Source: three-view drawing plus pictorial views. Frame: mm from the lowest corner of the part. Give positions to 0.01 mm unless a question says otherwise; leave off trailing zeros. Loops run counter-clockwise (first coordinate to the right, second up) from the corner with the lowest first, then second, coordinate; pieces in that order, holes last. Notation, with made-up numbers: M 49.25,-16 L 88.25,-16 A22 cw 88.25,-8 Z; hole C 42.5,23 d8. An arc over 180 degrees is marked long. Answer as a JSON object with one key per item and string values. Group by question number.
1) Section query D-D on x = 84.5. Return loops of the section in (y, z).
2) First-contact query: P1, Ø1, axis at y = 12.5, z = 3.5, coming from the -X side; P2, Ø3, axis at x = 51.6, y = 17.5, coming from the -Z side. Flat tips, straight axial feed; report the tip coordinate or a pass-through.
3) Ray query, L1, parallel to Y at x = 5, z = 4.5; L2, parallel to Y at x = 50.5, z = 4.5; L3, parallel to X at y = 17, z = 4.5. Return the intervals inside material, ascending.
4) Section query A-A on x = 51.6. Return loops of the section in (y, z).
5) Section query B-B on y = 52.5. Return loops of the section in (x, z), plus the area to 3 significant figures.
6) Section query C-C on z = 4.5. Count the separate pieces of the cut face and the enclosed holes in it, plus the area to 3 significant figures.
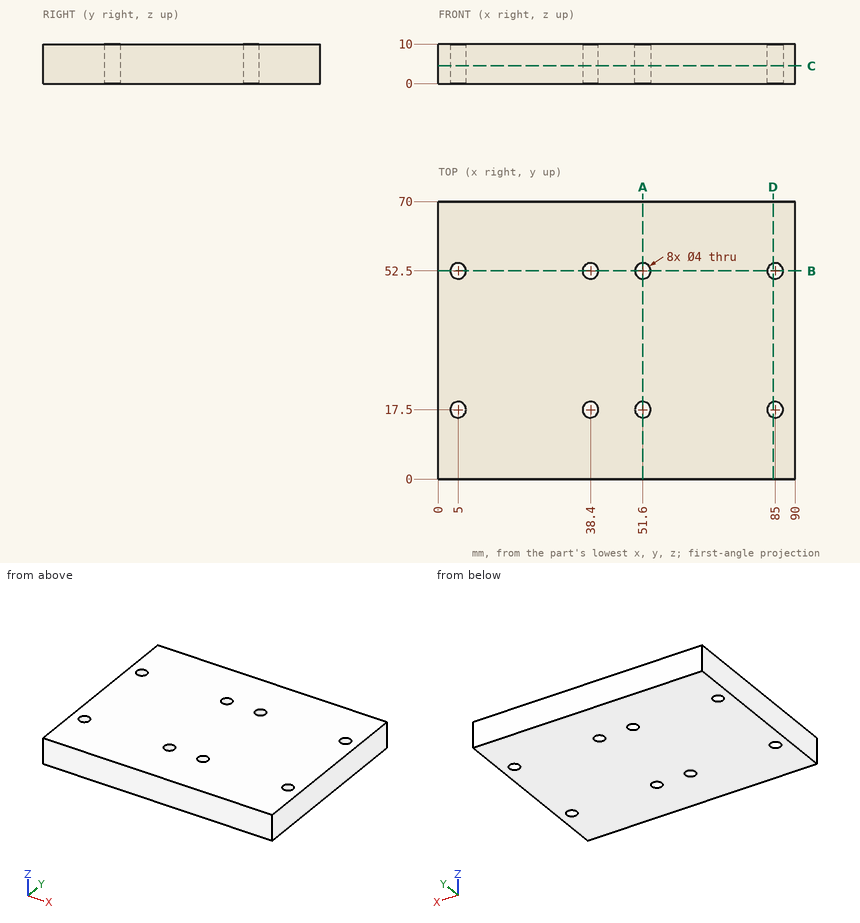
Output:
{
 "1": {"outline": "M 0,0 L 15.56,0 L 15.56,10 L 0,10 Z; M 19.44,0 L 50.56,0 L 50.56,10 L 19.44,10 Z; M 54.44,0 L 70,0 L 70,10 L 54.44,10 Z"},
 "2": {"P1": "stops at x = 0", "P2": "passes through"},
 "3": {"L1": "y = 0 to 15.5, 19.5 to 50.5, 54.5 to 70", "L2": "y = 0 to 15.83, 19.17 to 50.83, 54.17 to 70", "L3": "x = 0 to 3.06, 6.94 to 36.46, 40.34 to 49.66, 53.54 to 83.06, 86.94 to 90"},
 "4": {"outline": "M 0,0 L 15.5,0 L 15.5,10 L 0,10 Z; M 19.5,0 L 50.5,0 L 50.5,10 L 19.5,10 Z; M 54.5,0 L 70,0 L 70,10 L 54.5,10 Z"},
 "5": {"outline": "M 0,0 L 3,0 L 3,10 L 0,10 Z; M 7,0 L 36.4,0 L 36.4,10 L 7,10 Z; M 40.4,0 L 49.6,0 L 49.6,10 L 40.4,10 Z; M 53.6,0 L 83,0 L 83,10 L 53.6,10 Z; M 87,0 L 90,0 L 90,10 L 87,10 Z", "area": "740 mm^2"},
 "6": {"separate pieces": "1", "enclosed holes": "8", "area": "6,200 mm^2"}
}
